from build123d import *

# Parameters (mm, degrees)
SWEEP1_START        = -19.05
SWEEP1_DEPTH        = 38.1
BOSS_EXTRUDE1_START = -9.525
SKETCH4_R           = 3.175
BOSS_EXTRUDE1_DEPTH = 19.05
FILLET1_R           = 12.7


# Read off the part's stored shape, not the designer's step: Sweep1
with BuildPart() as part:
    # Sweep1 outline → Sweep1 (new body)
    with BuildSketch(Plane.XY.offset(SWEEP1_START)):
        Polygon((82.55, 28.575), (82.55, 47.625), (38.1, 47.625), (0, 9.525), (0, -9.525), (38.1, 28.575), align=None)
    extrude(amount=SWEEP1_DEPTH)

    # Sketch4 → Boss-Extrude1 (add)
    with BuildSketch(Plane(origin=(0, 0, 0), x_dir=(1, 0, 0), z_dir=(0, 1, 0)).offset(BOSS_EXTRUDE1_START)):
        with BuildLine():
            Line((0, 19.05), (-6.35, 19.05))
            ThreePointArc((-6.35, 19.05), (-25.4, 0), (-6.35, -19.05))
            Line((-6.35, -19.05), (0, -19.05))
            Line((0, -19.05), (0, 19.05))
        make_face()
        with Locations(Location((-12.7, 0, 0), (0, 0, 90))):
            Circle(SKETCH4_R, mode=Mode.SUBTRACT)
    extrude(amount=BOSS_EXTRUDE1_DEPTH)

    # Mirror4: part across plane


with BuildPart() as part_1:
    add(part.part)
    add(part.part.mirror(Plane(origin=(82.55, 0, 0), x_dir=(0, 0, 1), z_dir=(1, 0, 0))))

    # Fillet1
    fillet1_edges = [part_1.edges().sort_by_distance(p)[0] for p in [
        (38.1, 47.625, 0),
        (38.1, 28.575, 0),
        (127, 47.625, 0),
        (127, 28.575, 0),
    ]]
    fillet(fillet1_edges, radius=FILLET1_R)


solid = part_1.part
Geometry: final body of the model. Coordinates: model frame, mm. A direction names the side the tool comes from. Give positions to 0.01 mm unless a question says otherwise; leave off trailing zeros. Order: outer loops, then holes, each group sorted by start corner. A loop starts at its lowest first (then second) coordinate and runs counter-clockwise, first axis right, second up. Notation, with made-up numbers: (-23, -11) -> (0, -11) arc R18 ccw to (0, 0) -> close; hole circle Ø1 at (-2.5, 63). An arc over 180 degrees is marked (long way). Put each result on its own line as item: value.
Q1. Material intervals for L1, parallel to X at y = -2.75, z = 0 (3 decimals); L2, parallel to Y at x = 57, z = 9.5 (3 decimals); L3, parallel to X at y = -3.5, z = 0 (3 decimals), sorted ascending.
Here are the results:
L1: x = -25.4 to -15.875, -9.525 to 6.775, 158.325 to 174.625, 180.975 to 190.5
L2: y = 28.575 to 47.625
L3: x = -25.4 to -15.875, -9.525 to 6.025, 159.075 to 174.625, 180.975 to 190.5
Q2. Draft query along X for faces 1 (the face through (16.949, 7.424, -0.267)), 2 (the face through (17.431, 26.956, -0.267)), 3 (the face through (82, 29, -19.05)), 4 (the face through (-9.9, -0.1, -1.5)). Return one class per face: released by +X, released by -X, zero draft, split by the parting line, or undercut.
Here are the results:
face 1: undercut
face 2: released by -X
face 3: zero draft
face 4: undercut
Q3. Section A-A, the plane z = 0. Return loops of the section in (x, y) (3 decimals).
Here are the results:
outline: (-25.4, -9.525) -> (-15.875, -9.525) -> (-15.875, 9.525) -> (-25.4, 9.525) -> close; (-9.525, -9.525) -> (0, -9.525) -> (34.38, 24.855) arc R12.7 cw to (43.361, 28.575) -> (121.739, 28.575) arc R12.7 cw to (130.72, 24.855) -> (165.1, -9.525) -> (174.625, -9.525) -> (174.625, 9.525) -> (165.1, 9.525) -> (130.72, 43.905) arc R12.7 ccw to (121.739, 47.625) -> (43.361, 47.625) arc R12.7 ccw to (34.38, 43.905) -> (0, 9.525) -> (-9.525, 9.525) -> close; (180.975, -9.525) -> (190.5, -9.525) -> (190.5, 9.525) -> (180.975, 9.525) -> close
Q4. Section B-B, the plane y = 20.5. Return loops of the section in (x, z) (3 decimals).
Here are the results:
outline: (10.975, -19.05) -> (30.025, -19.05) -> (30.025, 19.05) -> (10.975, 19.05) -> close; (135.075, -19.05) -> (154.125, -19.05) -> (154.125, 19.05) -> (135.075, 19.05) -> close
Q5. Reachability of faces 5 (the face through (190.495, -0.133, -0.419)), 6 (the face through (-7, 9.525, 0)), 7 (the face through (126.535, 27.635, 0.267)), 8 (the face through (82, 47.625, 0)), 9 (the face through (172, 9.525, 0)) from +Z, -Z, +X, -X, +Y, -Y: full face, straight path, thin tool, end or side. Return the list, or none.
Here are the results:
face 5: +X, +Y, -Y
face 6: +Z, -Z, -X, +Y
face 7: +Z, -Z, -Y
face 8: +Z, -Z, +X, -X, +Y
face 9: +Z, -Z, +X, +Y
Q6. Section C-C, the plane x = 177.8. Return loops of the section in (y, z) (3 decimals).
Here are the results:
outline: (-9.525, -17.961) -> (9.525, -17.961) -> (9.525, -3.175) -> (-9.525, -3.175) -> close; (-9.525, 3.175) -> (9.525, 3.175) -> (9.525, 17.961) -> (-9.525, 17.961) -> close
Q7. Section D-D, the plane y = -4. Return loops of the section in (x, z) (3 decimals), then the cut area to 3 significant figures.
Here are the results:
outline: (-6.35, -19.05) -> (5.525, -19.05) -> (5.525, 19.05) -> (-6.35, 19.05) arc R19.05 ccw to start; (159.575, -19.05) -> (171.45, -19.05) arc R19.05 ccw to (171.45, 19.05) -> (159.575, 19.05) -> close; hole circle Ø6.35 at (-12.7, 0); hole circle Ø6.35 at (177.8, 0)
area: 1,980 mm^2
Q8. Pin query (flat end, axial travel): pin 1 (12 mm diameter, centred on y = 11, z = -8, fed in from -X); pin 2 (4 mm diameter, centred on x = 118.5, z = 7.5, fed in from -Y) (3 decimals); pin 3 (8 mm diameter, centred on y = 35, z = 8, fed in from -X) (3 decimals). Return the tip coordinate at first contact, or that it passes through.
Here are the results:
pin 1: stops at x = -25.27
pin 2: stops at y = 28.575
pin 3: stops at x = 21.475
